Model file for the job. Use its own axes, mm. Face numbers are marked on the shaded views. A direction names the side the tool comes from. Give positions to 0.01 mm unless a question says otherwise; leave off trailing zeros. Loops run counter-clockwise (first coordinate to the right, second up) from the corner with the lowest first, then second, coordinate; pieces in that order, holes last. Notation, with made-up numbers: (44.25, 64.5) - (83.25, 64.5) arc R27 ccw to (83.25, 92.5) - close; hole circle Ø9 at (-32.5, 67.5). An arc over 180 degrees is marked (long way). Use a Markdown table: item, result.
from build123d import *

# Parameters (mm, degrees)
EXTRUDE_1_DEPTH     = 12
SKETCH_2_R          = 5.5
CUT_EXTRUDE_1_DEPTH = 40.458839314
FILLET_1_R          = 5


with BuildPart() as part:
    # 草图1 → 凸台-拉伸1 (new, symmetric)
    with BuildSketch(Plane.XY):
        with BuildLine():
            Line((-33, 0), (33, 0))
            Line((33, 0), (33, 8))
            Line((33, 8), (18, 8))
            Line((18, 8), (18, 26))
            Line((18, 26), (13, 26))
            ThreePointArc((13, 26), (0, 13), (-13, 26))
            Line((-13, 26), (-18, 26))
            Line((-18, 26), (-18, 8))
            Line((-18, 8), (-33, 8))
            Line((-33, 8), (-33, 0))
        make_face()
    extrude(amount=EXTRUDE_1_DEPTH, both=True)

    # 草图2 → 切除-拉伸1 (cut, through all)
    with BuildSketch(Plane(origin=(0, 8, 0), x_dir=(1, 0, 0), z_dir=(0, 1, 0))):
        with Locations(Location((25, 0, 0), (0, 0, 180))):
            Circle(SKETCH_2_R)
        with Locations((-25, 0)):
            Circle(SKETCH_2_R)
    extrude(amount=-CUT_EXTRUDE_1_DEPTH, mode=Mode.SUBTRACT)

    # 圆角1
    fillet_1_edges = [part.edges().sort_by_distance(p)[0] for p in [
        (33, 4, -12),
        (-33, 4, -12),
        (-33, 4, 12),
        (33, 4, 12),
    ]]
    fillet(fillet_1_edges, radius=FILLET_1_R)


solid = part.part
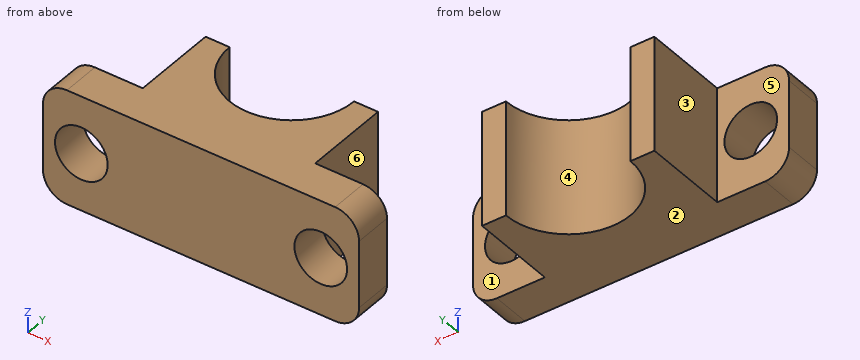
(1) 3-axis set-ups, long thin cutter, end or side, ignore diameter. For the marked faces 1, 2 and 3: which of +Z, -Z, +X, -X, +Y, -Y reach the whole face in a straight line?
Computed:
| item | result |
|---|---|
| face 1 | +Z, -Z, +X, +Y |
| face 2 | -Z, +X, -X, +Y, -Y |
| face 3 | +Z, -Z, -X, +Y |
(2) Slice it at D-D, the plane z = -8. Write the cut outline in (x, y), plus the area to 3 significant figures.
Computed:
| item | result |
|---|---|
| outline | (-32.9, 0) - (32.9, 0) - (32.9, 8) - (18, 8) - (18, 26) - (13, 26) arc R13 cw to (-13, 26) - (-18, 26) - (-18, 8) - (-32.9, 8) - close |
| area | 909 mm² |
(3) Mould opens along X. For the marked faces 4, 5 and 6 say: pulls with the +X half, pulls with the -X half, needs draft (parallel to the pull), parting line crosses it, or undercut.
Computed:
| item | result |
|---|---|
| face 4 | undercut |
| face 5 | needs draft |
| face 6 | pulls with the +X half |
(4) Slice it at C-C, the plane y = 20.25. Write the cut outline in (x, z), plus the area to 3 significant figures.
Computed:
| item | result |
|---|---|
| outline | (-18, -12) - (-11.66, -12) - (-11.66, 12) - (-18, 12) - close; (11.66, -12) - (18, -12) - (18, 12) - (11.66, 12) - close |
| area | 304 mm² |
(5) Drill centre lines: probe 1 along Z at (x, y) = (25, 3.5); probe 2 along X at (y, z) = (5, -4.75); probe 3 along Y at (x, z) = (24, 9.75). Where is each one in solid material? Low to high. Write a range as [from, to].
Computed:
| item | result |
|---|---|
| probe 1 | [-12, -5.5], [5.5, 12] |
| probe 2 | [-33, -27.77], [-22.23, 22.23], [27.77, 33] |
| probe 3 | [0, 8] |
(6) Slice it at B-B, the plane x = -25. Write the cut outline in (y, z).
Computed:
| item | result |
|---|---|
| outline | (0, -12) - (8, -12) - (8, -5.5) - (0, -5.5) - close; (0, 5.5) - (8, 5.5) - (8, 12) - (0, 12) - close |
(7) Slice it at A-A, the plane z = 0. Write the cut outline in (x, y).
Computed:
| item | result |
|---|---|
| outline | (-33, 0) - (-30.5, 0) - (-30.5, 8) - (-33, 8) - close; (-19.5, 0) - (19.5, 0) - (19.5, 8) - (18, 8) - (18, 26) - (13, 26) arc R13 cw to (-13, 26) - (-18, 26) - (-18, 8) - (-19.5, 8) - close; (30.5, 0) - (33, 0) - (33, 8) - (30.5, 8) - close |
(8) Pin check, flat tips, straight feed: P1, Ø12, axis at x = 29, z = 4.5, coming from the +Y side; P2, Ø9, axis at y = 15.5, z = 0.5, coming from the -X side; P3, Ø2, axis at x = 13.5, z = -4, coming from the -Y side; P4, Ø6, axis at x = -24.5, z = -0.5, coming from the +Y side. Stop position of each tip, or through.
Computed:
| item | result |
|---|---|
| P1 | y = 8 |
| P2 | x = -18 |
| P3 | y = 0 |
| P4 | through |
